from build123d import *

# Parameters (mm, degrees)
RESSALTO_EXTRUS_O1_DEPTH = 2.5
FILETE1_R                = 0.1


with BuildPart() as part:
    # Esboço1 → Ressalto-extrusão1 (new body)
    with BuildSketch(Plane.XY):
        with BuildLine():
            Line((-88.734374253, 18.21347197), (-88.734374253, 20.71347197))
            Line((-88.734374253, 20.71347197), (-81.846885596, 20.71347197))
            ThreePointArc((-81.846885596, 20.71347197), (-95.734374253, 19.46347197), (-81.846885596, 18.21347197))
            Line((-81.846885596, 18.21347197), (-88.734374253, 18.21347197))
        make_face()
    extrude(amount=RESSALTO_EXTRUS_O1_DEPTH)

    # Filete1
    filete1_edges = [part.edges().sort_by_distance(p)[0] for p in [
        (-85.290629924, 18.21347197, 2.5),
        (-88.734374253, 19.46347197, 2.5),
        (-85.290629924, 20.71347197, 2.5),
        (-88.734374253, 19.46347197, 0),
        (-85.290629924, 18.21347197, 0),
        (-95.734374253, 19.46347197, 0),
        (-85.290629924, 20.71347197, 0),
        (-88.734374253, 20.71347197, 1.25),
        (-88.734374253, 18.21347197, 1.25),
        (-81.846885596, 18.21347197, 1.25),
        (-81.846885596, 20.71347197, 1.25),
        (-95.734374253, 19.46347197, 2.5),
    ]]
    fillet(filete1_edges, radius=FILETE1_R)


solid = part.part
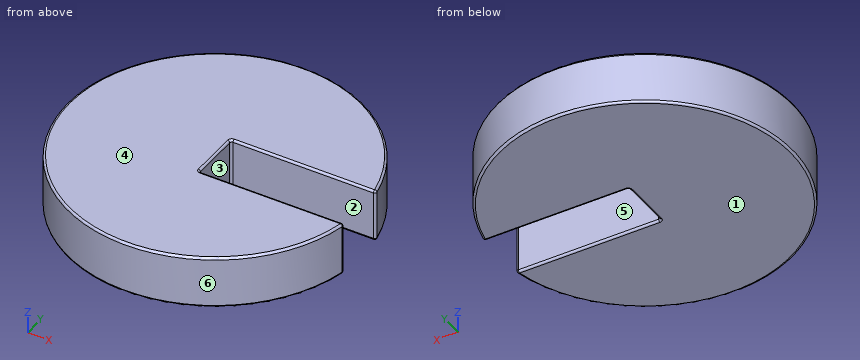
Here's how the part is built. I have some questions about the finished solid (model axes, mm). Face numbers are marked on the shaded views. A direction names the side the tool comes from. Round coordinates to 2 decimals unless told otherwise and drop trailing zeros. Loops run counter-clockwise (first coordinate to the right, second up) from the corner with the lowest first, then second, coordinate; pieces in that order, holes last. Notation, with made-up numbers: M 25,9.5 L 76,9.5 A25 ccw 76,33.5 Z; hole C 47,52 d5. An arc over 180 degrees is marked long. Write each question's results on one line, items separated by ' | '. Start each with the question number.
(1) If I drill on probe 1 along Y at (x, z) = (-88.5, 0.35); probe 2 along Y at (x, z) = (-86.25, 1.4); probe 3 along X at (y, z) = (21, 0.6), over which ranges is the centre line in solid material (lowest first)? Write a range as from..to.
(2) Thinking about a two-plate mould opening in Y: for the marked faces 3, 4, 5 and 6, which applies, pulls with the +Y half, pulls with the -Y half, needs draft (parallel to the pull), parting line crosses it, or undercut?
(3) I want a section at A-A (z = 1.45). Please give me the cut outline in (x, y), then the cut area to 3 significant figures.
(4) Will these pins go through, and if not, where does the flat tip stop? P1, Ø1.5, axis at y = 17, z = 0.5, coming from the +X side; P2, Ø0.7, axis at x = -84, z = 0.5, coming from the -Y side; P3, Ø1.2, axis at x = -85.5, z = 1.5, coming from the +Y side.
(5) On a 3-axis mill with a long thin cutter (end or side, diameter ignored), from which of +Z, -Z, +X, -X, +Y, -Y can I reach the whole of each face in a straight line? I mean the marked faces 1 and 2. Say none if no direction works.
Solved:
1) probe 1: y = 12.47..18.21, 20.71..26.46 | probe 2: y = 12.92..18.21, 20.71..26.01 | probe 3: x = -95.56..-81.91
2) face 3: undercut | face 4: needs draft | face 5: undercut | face 6: parting line crosses it
3) outline: M -88.73,18.31 L -88.73,20.61 A0.1 cw -88.63,20.71 L -81.97,20.71 A0.1 ccw -81.87,20.83 A7 ccw long -81.87,18.09 A0.1 ccw -81.97,18.21 L -88.63,18.21 A0.1 cw Z | area: 137 mm²
4) P1: stops at x = -81.95 | P2: stops at y = 14.01 | P3: stops at y = 25.95
5) face 1: -Z, +X, -X, +Y, -Y | face 2: +Z, -Z, +X
